from build123d import *

# Parameters (mm, degrees)
SKETCH1_W           = 25
SKETCH1_H           = 25
SKETCH1_W_2         = 21
SKETCH1_H_2         = 21
BOSS_EXTRUDE1_DEPTH = 275
SKETCH2_R           = 2
BOSS_EXTRUDE2_DEPTH = 30


with BuildPart() as part:
    # Sketch1 → Boss-Extrude1 (new body)
    with BuildSketch(Plane.XY):
        Rectangle(SKETCH1_W, SKETCH1_H)
        Rectangle(SKETCH1_W_2, SKETCH1_H_2, mode=Mode.SUBTRACT)
    extrude(amount=BOSS_EXTRUDE1_DEPTH)

    # Sketch2 → Boss-Extrude2 (add)
    with BuildSketch(Plane.XY.offset(136.5)):
        with BuildLine():
            Line((12.5, -12.5), (12.5, -13.285898385))
            ThreePointArc((12.5, -13.285898385), (10.5, -20.75), (8.5, -13.285898385))
            Line((8.5, -13.285898385), (8.5, -12.5))
            Line((8.5, -12.5), (12.5, -12.5))
        make_face()
        with Locations((10.5, -16.75)):
            Circle(SKETCH2_R, mode=Mode.SUBTRACT)
    extrude(amount=-BOSS_EXTRUDE2_DEPTH)


solid = part.part
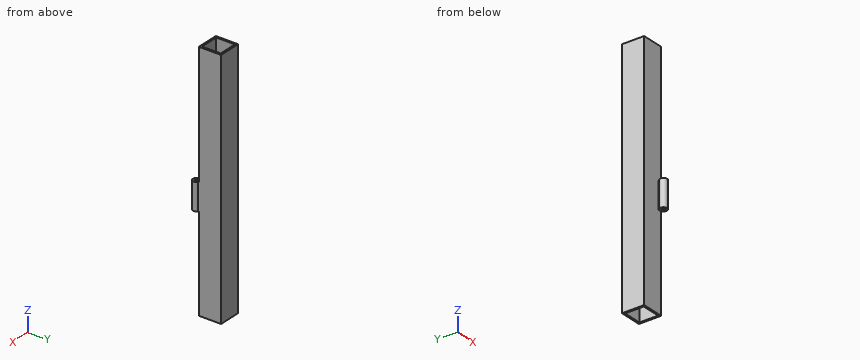
Check sheet for the modelled part. Datum: model origin and axes. Units: mm. Coordinates: 2 decimals unless noted, no trailing zeros. Write each loop counter-clockwise with the first axis right and the second up, starting at its lowest first coordinate (ties: lowest second). Pieces come first, ordered by that corner, then holes.
Item 1: Cross-section at A-A on y = 4.5. Record the boundary of the cut face in (x, z), then the cut area to 3 significant figures.
Numbers:
outline: (-12.5, 0) - (-10.5, 0) - (-10.5, 275) - (-12.5, 275) - close; (10.5, 0) - (12.5, 0) - (12.5, 275) - (10.5, 275) - close
area: 1,100 mm2
Item 2: Depth check by flat-ended pin: pin 1 Ø5 at (y, z) = (5.5, 104) entering from +X; pin 2 Ø1.5 at (x, z) = (9.5, 117.5) entering from -Y; pin 3 Ø3.5 at (x, y) = (10.5, -16.75) entering from -Z; pin 4 Ø8 at (x, z) = (-8.5, 41) entering from -Y. Enter the tip coordinate at first touch or a pass-through.
Numbers:
pin 1: stops at x = 12.5
pin 2: stops at y = -20.74
pin 3: passes through
pin 4: stops at y = -12.5
Item 3: Scan lines: probe 1 along Y at (x, z) = (-6, 58); probe 2 along X at (y, z) = (-16, 127). Record each from-to range of solid material in increasing order.
Numbers:
probe 1: y = -12.5 to -10.5, 10.5 to 12.5
probe 2: x = 6.57 to 8.65, 12.35 to 14.43
Item 4: Cross-section at B-B on z = 122.5. Record the boundary of the cut face in (x, y), then the cut area to 3 significant figures.
Numbers:
outline: (-12.5, -12.5) - (8.5, -12.5) - (8.5, -13.29) arc R4 ccw (long way) to (12.5, -13.29) - (12.5, 12.5) - (-12.5, 12.5) - close; hole (-10.5, -10.5) - (10.5, -10.5) - (10.5, 10.5) - (-10.5, 10.5) - close; hole circle Ø4 at (10.5, -16.75)
area: 223 mm2
Item 5: Cross-section at C-C on z = 250. Record the boundary of the cut face in (x, y).
Numbers:
outline: (-12.5, -12.5) - (12.5, -12.5) - (12.5, 12.5) - (-12.5, 12.5) - close; hole (-10.5, -10.5) - (10.5, -10.5) - (10.5, 10.5) - (-10.5, 10.5) - close
